For this review, take the finished solid that the model builds, in its own axes (mm). A direction names the side the tool comes from. Coordinates: 2 decimals unless noted, no trailing zeros. Loops run counter-clockwise (first coordinate to the right, second up) from the corner with the lowest first, then second, coordinate; pieces in that order, holes last. Notation, with made-up numbers: (-8.75, 30.25) -> (30.25, 30.25) arc R6 cw to (30.25, 41.25) -> close; hole circle Ø2 at (40.5, 40.25). An arc over 180 degrees is marked (long way). One line per item, written item: value.
from build123d import *

# Parameters (mm, degrees)
SKETCH1_R               = 3
BOSS_EXTRUDE1_DEPTH     = 7.2
CUT_EXTRUDE1_REACH      = 9.2
SKETCH2_R               = 1.5
SKETCH3_W               = 2.1
SKETCH3_H               = 2.4
CUT_EXTRUDE2_DEPTH      = 4
CUT_EXTRUDE2_DEPTH_BACK = 4
CHAMFER1_SIZE           = 0.2


with BuildPart() as part:
    # Sketch1 → Boss-Extrude1 (new body)
    with BuildSketch(Plane(origin=(0, 0, 0), x_dir=(1, 0, 0), z_dir=(0, 1, 0))):
        Circle(SKETCH1_R)
    extrude(amount=BOSS_EXTRUDE1_DEPTH)

    # Sketch2 → Cut-Extrude1 (cut, up to next)
    with BuildSketch(Plane(origin=(0, 7.2, 0), x_dir=(1, 0, 0), z_dir=(0, 1, 0)), mode=Mode.PRIVATE) as cut_extrude1_sk1:
        Circle(SKETCH2_R)
    cut_extrude1_tool1 = extrude(cut_extrude1_sk1.sketch, amount=-CUT_EXTRUDE1_REACH, mode=Mode.PRIVATE) & part.part
    add(cut_extrude1_tool1.solids().sort_by_distance((0, 7.2, 0))[0], mode=Mode.SUBTRACT)

    # Sketch3 → Cut-Extrude2 (cut, two sides)
    with BuildSketch(Plane.XY) as cut_extrude2_sk:
        with Locations((1.95, 3.2)):
            Rectangle(SKETCH3_W, SKETCH3_H)
    extrude(amount=CUT_EXTRUDE2_DEPTH, mode=Mode.SUBTRACT)
    extrude(cut_extrude2_sk.sketch, amount=-CUT_EXTRUDE2_DEPTH_BACK, mode=Mode.SUBTRACT)

    # Chamfer1
    chamfer1_edges = [part.edges().sort_by_distance(p)[0] for p in [
        (-1.5, 7.2, 0),
    ]]
    chamfer(chamfer1_edges, length=CHAMFER1_SIZE)


solid = part.part
1. Take a section at A-A, the plane z = 0. Give the boundary of the cut face in (x, y), and give its area (3 significant figures).
Return value:
outline: (-3, 0) -> (-1.5, 0) -> (-1.5, 7) -> (-1.7, 7.2) -> (-3, 7.2) -> close; (1.5, 0) -> (3, 0) -> (3, 2) -> (1.5, 2) -> close; (1.5, 4.4) -> (3, 4.4) -> (3, 7.2) -> (1.7, 7.2) -> (1.5, 7) -> close
area: 18.0 mm2
2. For faces 1 (the flat face through (0.9, 3, 2)), 2 (the flat face through (1.3, 0, 1.3)), list the 3-axis set-ups (+Z, -Z, +X, -X, +Y, -Y) from which the entire face can be reached by the end or side of a thin tool; tool diameter is ignored.
Return value:
face 1: +Z, -Z, +X
face 2: +Z, -Z, +X, -X, -Y
3. Take a section at D-D, the plane x = 2.35. Give the boundary of the cut face in (y, z).
Return value:
outline: (0, -1.86) -> (2, -1.86) -> (2, 1.86) -> (0, 1.86) -> close; (4.4, -1.86) -> (7.2, -1.86) -> (7.2, 1.86) -> (4.4, 1.86) -> close
4. Insertion check: pin 1 Ø2 at (y, z) = (6.5, 2) entering from +X; pin 2 Ø0.5 at (y, z) = (3, 2) entering from +X; pin 3 Ø1.8 at (y, z) = (2.5, -2) entering from +X. Each pin has a flat end and moves straight along its axis. Give the tip position at first contact, or say it passes through.
Return value:
pin 1: stops at x = 2.83
pin 2: stops at x = 0.9
pin 3: stops at x = 2.73
5. The part is to be moulded in two halves that separate along X. For faces 3 (the flat face through (2, 4.4, 0)), 4 (the flat face through (0.9, 3, -2)), 5 (the cylindrical face through (-3, 4, 0)), 6 (the cylindrical face through (-1.5, 3.55, -0.07)), say which applies: pulls with the +X half, pulls with the -X half, needs draft (parallel to the pull), parting line crosses it, or undercut.
Return value:
face 3: needs draft
face 4: pulls with the +X half
face 5: parting line crosses it
face 6: undercut
6. Take a section at C-C, the plane y = 0.5. Give the boundary of the cut face in (x, z).
Return value:
outline: circle Ø6 at (0, 0); hole circle Ø3 at (0, 0)
7. To check wall thickness, follow probe 1 along Y at (x, z) = (1.9, -0.4); probe 2 along Z at (x, y) = (0, 5.5). State the ranges of each line that lie inside material, in increasing order. Write a range as from..to.
Return value:
probe 1: y = 0..2, 4.4..7.2
probe 2: z = -3..-1.5, 1.5..3
8. Take a section at B-B, the plane x = 0. Give the boundary of the cut face in (y, z).
Return value:
outline: (0, -3) -> (7.2, -3) -> (7.2, -1.7) -> (7, -1.5) -> (0, -1.5) -> close; (0, 1.5) -> (7, 1.5) -> (7.2, 1.7) -> (7.2, 3) -> (0, 3) -> close
